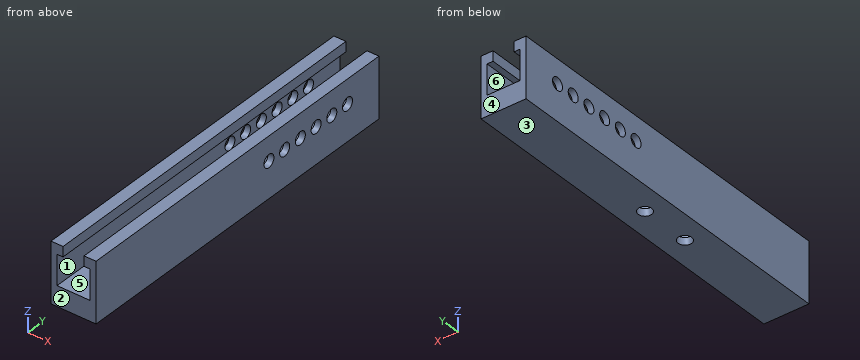
```python
from build123d import *

# Parameters (mm, degrees)
F1_DEPTH       = 90
F3_D           = 6.7564
F3_CBORE_D     = 10
F3_CBORE_DEPTH = 6.35
F4_R           = 3.175
F5_DEPTH       = 25
F7_D           = 6.7564
F7_CBORE_D     = 10
F7_CBORE_DEPTH = 6.35


with BuildPart() as f1:
    # F0 (on Front) → F1 (new body, symmetric)
    with BuildSketch(Plane.XZ):
        Polygon((-11.25, -10), (0, -10), (11.25, -10), (11.25, 20), (5.25, 20), (5.25, 15), (8.25, 15), (8.25, 0), (5.25, 0), (0, 0), (-5.25, 0), (-8.25, 0), (-8.25, 15), (-5.25, 15), (-5.25, 20), (-11.25, 20), align=None)
    extrude(amount=F1_DEPTH, both=True)

    # F3 (through all)
    with Locations(Plane.XY):
        with Locations((0, 0)):
            CounterBoreHole(F3_D / 2, F3_CBORE_D / 2, F3_CBORE_DEPTH)

    # F4 (on face) → F5 (cut)
    with BuildSketch(Plane.YZ.offset(11.25)):
        with Locations((40, 8)):
            Circle(F4_R)
        with Locations((50, 8)):
            Circle(F4_R)
        with Locations((60, 8)):
            Circle(F4_R)
        with Locations((30, 8)):
            Circle(F4_R)
        with Locations((20, 8)):
            Circle(F4_R)
        with Locations((70, 8)):
            Circle(F4_R)
    extrude(amount=-F5_DEPTH, mode=Mode.SUBTRACT)

    # F7 (through all)
    with Locations(Plane.XY):
        with Locations((0, -25.4)):
            CounterBoreHole(F7_D / 2, F7_CBORE_D / 2, F7_CBORE_DEPTH)


solid = f1.part
```
Could you check a few things on this model? Use its own coordinates, in mm. Face numbers are marked on the shaded views. A direction names the side the tool comes from. Give positions to 0.01 mm unless a question says otherwise; leave off trailing zeros. Order: outer loops, then holes, each group sorted by start corner. A loop starts at its lowest first (then second) coordinate and runs counter-clockwise, first axis right, second up.
Q1. If I drill on line 1 along Z through (x, y) = (9.75, 60) (3 decimals); line 2 along X through (y, z) = (56, 8); line 3 along Y through (x, z) = (-0.75, -6.75), over which ranges is the centre line in solid material (lowest first)?
Q2. I'm going to push a flat-ended pin straight in: P1, Ø5, axis at x = 5, z = 4, coming from the +Y side. Where does the tip first touch, or does it pass through?
Q3. Suppose I cut it at B-B, the plane y = 20. Write out the boundary of the cut face in (x, z) (3 decimals).
Q4. We'd pull the mould along Z, two halves only. Please class the marked faces 3, 4, 5 and 6: +Z half, -Z half, draft (parallel to the pull), parting line (faces both ways), or undercut.
Q5. For the marked faces 1 and 2, which set-ups out of +Z, -Z, +X, -X, +Y, -Y let a thin tool reach every point of the face, with its end or its side?
Q6. Suppose I cut it at D-D, the plane y = -25.4. Write out the boundary of the cut face in (x, z).
Q7. Suppose I cut it at A-A, the plane x = 0. Write out the boundary of the cut face in (y, z).
Q8. Suppose I cut it at C-C, the plane z = 13.25. Write out the boundary of the cut face in (x, y).
Solution:
1. line 1: z = -10 to 4.825, 11.175 to 20
1. line 2: x = -11.25 to -8.25, 8.25 to 11.25
1. line 3: y = -90 to -28.69, -22.11 to -3.29, 3.29 to 90
2. P1: passes through
3. outline: (-11.25, -10) - (11.25, -10) - (11.25, 4.825) - (8.25, 4.825) - (8.25, 0) - (-8.25, 0) - (-8.25, 4.825) - (-11.25, 4.825) - close; (-11.25, 11.175) - (-8.25, 11.175) - (-8.25, 15) - (-5.25, 15) - (-5.25, 20) - (-11.25, 20) - close; (5.25, 15) - (8.25, 15) - (8.25, 11.175) - (11.25, 11.175) - (11.25, 20) - (5.25, 20) - close
4. face 3: -Z half
4. face 4: draft
4. face 5: undercut
4. face 6: undercut
5. face 1: +Y, -Y
5. face 2: +Z, -Z, +X, -X, -Y
6. outline: (-11.25, -10) - (-3.38, -10) - (-3.38, -6.35) - (-5, -6.35) - (-5, 0) - (-8.25, 0) - (-8.25, 15) - (-5.25, 15) - (-5.25, 20) - (-11.25, 20) - close; (3.38, -10) - (11.25, -10) - (11.25, 20) - (5.25, 20) - (5.25, 15) - (8.25, 15) - (8.25, 0) - (5, 0) - (5, -6.35) - (3.38, -6.35) - close
7. outline: (-90, -10) - (-28.78, -10) - (-28.78, -6.35) - (-30.4, -6.35) - (-30.4, 0) - (-90, 0) - close; (-22.02, -10) - (-3.38, -10) - (-3.38, -6.35) - (-5, -6.35) - (-5, 0) - (-20.4, 0) - (-20.4, -6.35) - (-22.02, -6.35) - close; (3.38, -10) - (90, -10) - (90, 0) - (5, 0) - (5, -6.35) - (3.38, -6.35) - close
8. outline: (-11.25, -90) - (-8.25, -90) - (-8.25, 90) - (-11.25, 90) - close; (8.25, -90) - (11.25, -90) - (11.25, 90) - (8.25, 90) - close
